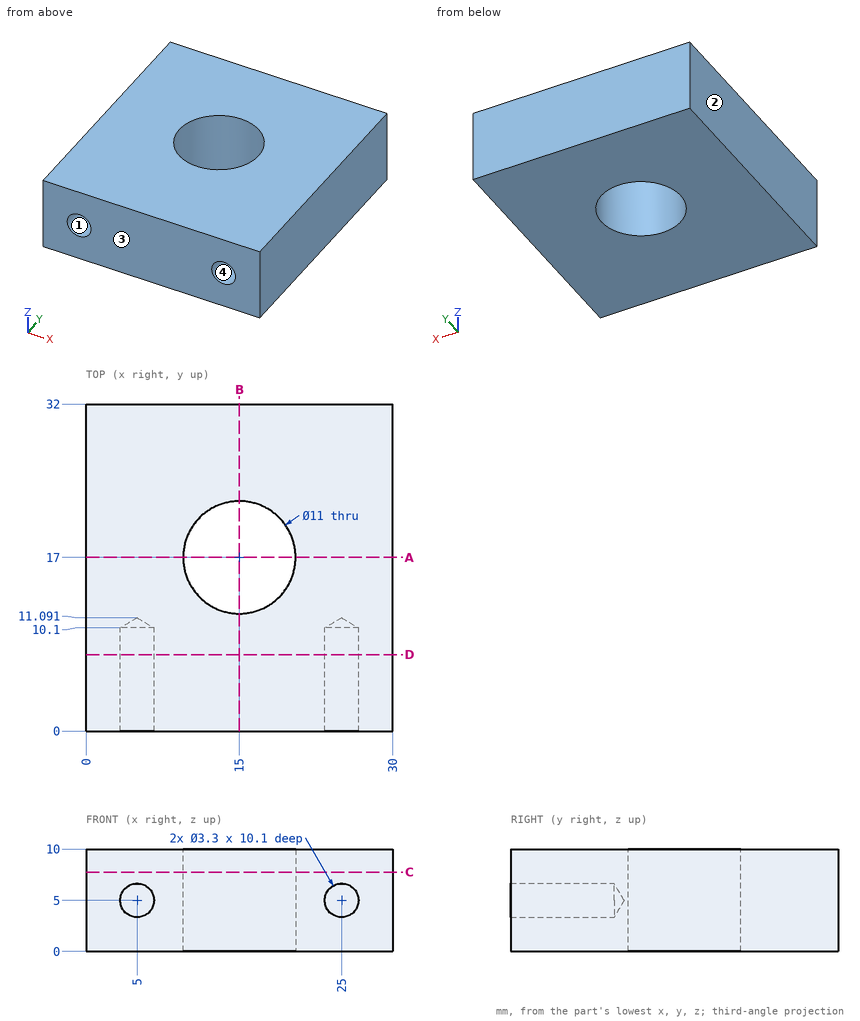
Source: three-view drawing plus pictorial views. Frame: mm from the lowest corner of the part. Give positions to 0.01 mm unless a question says otherwise; leave off trailing zeros. Loops run counter-clockwise (first coordinate to the right, second up) from the corner with the lowest first, then second, coordinate; pieces in that order, holes last. Notation, with made-up numbers: (23, 77) -> (67, 77) arc R34 cw to (67, 112) -> close; hole circle Ø9 at (53.25, 63). An arc over 180 degrees is marked (long way). Put each result on its own line as item: value. Start each with the question number.
1) Cut plane C-C (z = 7.75). Return loops of the section in (x, y), then the cut area to 3 significant figures.
2) Draft query along X for the marked faces 1, 2, 3 and 4. Return one class per face: released by +X, released by -X, zero draft, split by the parting line, or undercut.
3) Cut plane A-A (y = 17). Return loops of the section in (x, z).
4) Cut plane D-D (y = 7.5). Return loops of the section in (x, z).
5) Contact query for flat-ended pins moving along their axis: P1, Ø2.5, axis at x = 25, z = 5, coming from the -Y side; P2, Ø6, axis at y = 23.5, z = 3, coming from the -X side. Output: stop coordinate, or through.
6) Cut plane B-B (x = 15). Return loops of the section in (y, z), then the cut area to 3 significant figures.
7) Material intervals for probe 1 along X at (y, z) = (5, 5); probe 2 along X at (y, z) = (14.5, 9); probe 3 along Z at (x, y) = (25, 5.75), sorted ascending.
Results are:
1. outline: (0, 0) -> (30, 0) -> (30, 32) -> (0, 32) -> close; hole circle Ø11 at (15, 17)
1. area: 865 mm2
2. face 1: undercut
2. face 2: released by -X
2. face 3: zero draft
2. face 4: undercut
3. outline: (0, 0) -> (9.5, 0) -> (9.5, 10) -> (0, 10) -> close; (20.5, 0) -> (30, 0) -> (30, 10) -> (20.5, 10) -> close
4. outline: (0, 0) -> (30, 0) -> (30, 10) -> (0, 10) -> close; hole circle Ø3.3 at (5, 5); hole circle Ø3.3 at (25, 5)
5. P1: stops at y = 10.34
5. P2: stops at x = 0
6. outline: (0, 0) -> (11.5, 0) -> (11.5, 10) -> (0, 10) -> close; (22.5, 0) -> (32, 0) -> (32, 10) -> (22.5, 10) -> close
6. area: 210 mm2
7. probe 1: x = 0 to 3.35, 6.65 to 23.35, 26.65 to 30
7. probe 2: x = 0 to 10.1, 19.9 to 30
7. probe 3: z = 0 to 3.35, 6.65 to 10
